from build123d import *

# Parameters (mm, degrees)
SKETCH_R     = 15
SKETCH002_R  = 7.5
SKETCH001_R  = 15
SKETCH004_R  = 1.75
POCKET_DEPTH = 18


with BuildPart() as part:
    # Sketch → Loft section 0
    with BuildSketch(Plane.XY):
        with Locations((-60, 0)):
            Circle(SKETCH_R)
    # Sketch002 → Loft section 1
    with BuildSketch(Plane.YZ):
        with Locations((0, 34.505207)):
            Circle(SKETCH002_R)
    # Sketch001 → Loft section 2
    with BuildSketch(Plane.XY):
        with Locations((60, 0)):
            Circle(SKETCH001_R)
    loft()

    # Sketch004 → Pocket (cut)
    with BuildSketch(Plane.XY):
        with Locations((-52.5, 0)):
            Circle(SKETCH004_R)
        with Locations((52.5, 0)):
            Circle(SKETCH004_R)
    extrude(amount=POCKET_DEPTH, mode=Mode.SUBTRACT)


solid = part.part
Can you work these out from the model? Positions are in its coordinate system, mm. A direction names the side the tool comes from. Round coordinates to 2 decimals unless told otherwise and drop trailing zeros. Use one line per item in the form item = value. Start each with the question number.
Q1. Imagine slicing it at A-A (z = 12). Count the separate pieces of the cut face and the enclosed holes in it, then the cut area to 3 significant figures.
Q2. Which directions (+Z, -Z, +X, -X, +Y, -Y) give clear straight access to the entire face, cutting with the end or side of a thin tool? Please do faces 1 (the face through (-50.883, -0.67, 8.874)), 2 (the face through (60, -1, 0)).
Q3. I'm going to push flat-ended pins straight in: P1, Ø2, axis at y = -5, z = 16.5, coming from the +X side; P2, Ø1, axis at y = 3.5, z = 13, coming from the -X side; P3, Ø3, axis at y = 6.5, z = 13, coming from the +X side. Where does each tip first touch, or does it pass through?
Q4. We'd pull the mould along X, two halves only. Please class faces 3 (the face through (-60, -1, 0)), 4 (the face through (52, 0, 18)): +X half, -X half, draft (parallel to the pull), parting line (faces both ways), or undercut.
Q5. If I drill on probe 1 along X at (y, z) = (1.5, 10); probe 2 along X at (y, z) = (-9, 9); probe 3 along X at (y, z) = (4.5, 12.5), over which ranges is the centre line in solid material (lowest first)? Write a range as [from, to].
Worked out:
q1.separate_pieces = 2
q1.enclosed_holes = 2
q1.area = 1,140 mm^2
q2.face_1 = -Z
q2.face_2 = -Z, +X, -X, +Y, -Y
q3.P1 = 58.37
q3.P2 = -62.31
q3.P3 = 62.13
q4.face_3 = draft
q4.face_4 = undercut
q5.probe_1 = [-65.37, -53.4], [-51.6, -35.82], [35.82, 51.6], [53.4, 65.37]
q5.probe_2 = [-62.56, -41.11], [41.11, 62.56]
q5.probe_3 = [-61.89, -34.15], [34.15, 61.89]
